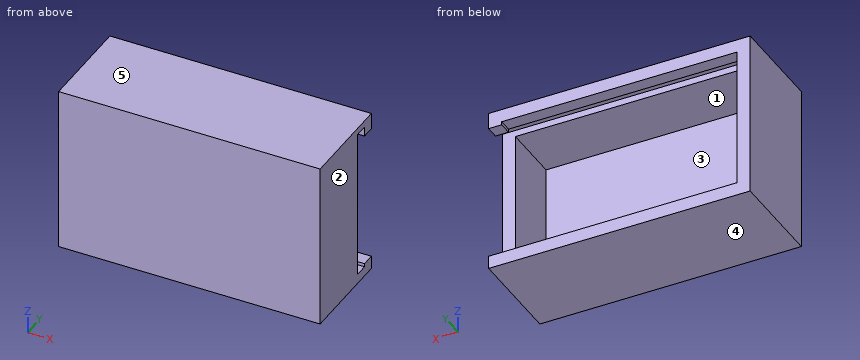
from build123d import *

# Parameters (mm, degrees)
SKETCH1_W           = 40
SKETCH1_H           = 25.5
BOSS_EXTRUDE1_DEPTH = 15
SHELL1_T            = -2
SKETCH2_W           = 21
SKETCH2_H           = 4
CUT_EXTRUDE1_DEPTH  = 2
SKETCH3_W           = 23.01
SKETCH3_H           = 2
CUT_EXTRUDE2_DEPTH  = 38


with BuildPart() as part:
    # Sketch1 → Boss-Extrude1 (new body)
    with BuildSketch(Plane(origin=(0, 0, 0), x_dir=(1, 0, 0), z_dir=(0, 1, 0))):
        Rectangle(SKETCH1_W, SKETCH1_H)
    extrude(amount=BOSS_EXTRUDE1_DEPTH)

    # Shell1
    shell1_openings = [part.faces().sort_by_distance(p)[0] for p in [
        (0, 15, 0),
    ]]
    offset(amount=SHELL1_T, openings=shell1_openings, kind=Kind.INTERSECTION)

    # Sketch2 → Cut-Extrude1 (cut)
    with BuildSketch(Plane(origin=(20, 0, 0), x_dir=(0, 0, -1), z_dir=(1, 0, 0))):
        with Locations((0.25, 13)):
            Rectangle(SKETCH2_W, SKETCH2_H)
    extrude(amount=-CUT_EXTRUDE1_DEPTH, mode=Mode.SUBTRACT)

    # Sketch3 → Cut-Extrude2 (cut)
    with BuildSketch(Plane(origin=(20, 0, 0), x_dir=(0, 0, -1), z_dir=(1, 0, 0))):
        with Locations((-0.245, 12)):
            Rectangle(SKETCH3_W, SKETCH3_H)
    extrude(amount=-CUT_EXTRUDE2_DEPTH, mode=Mode.SUBTRACT)


solid = part.part
Part model, mm, in its own coordinate system. Face numbers are marked on the shaded views. A direction names the side the tool comes from. Coordinates: 2 decimals unless noted, no trailing zeros. Loops run counter-clockwise (first coordinate to the right, second up) from the corner with the lowest first, then second, coordinate; pieces in that order, holes last. Notation, with made-up numbers: (-37.5, -14.75) -> (-18.5, -14.75) arc R20 cw to (-18.5, 5.25) -> close; hole circle Ø2 at (-28.75, 38). An arc over 180 degrees is marked (long way). Use a Markdown table: item, result. Add a question column.
Item 1: Band-saw the part on A-A on y = 6.25. Write the cut outline in (x, z), plus the area to 3 significant figures.
Item 2: Pull direction Z, two halves, no side cores. Call the marked faces 3, 4 and 5: +Z half, -Z half, draft (parallel to the pull), parting line (faces both ways), or undercut.
Item 3: Band-saw the part on C-C on x = -15. Write the cut outline in (y, z), plus the area to 4 significant figures.
Item 4: Which spindle directions (+Z, -Z, +X, -X, +Y, -Y) get a long thin tool onto all of the face, cutting with end or side? Do the marked faces 1 and 2. Say none if no direction does.
Item 5: Flat gauge pin, fed straight in: P1, Ø7, axis at x = -6, z = -3.5, coming from the +Y side. Where does the tip first touch, or does it go through?
Item 6: Probe probe 1 along Z at (x, y) = (3.5, 4); probe 2 along X at (y, z) = (3.75, 5); probe 3 along Y at (x, z) = (10.5, -9.75). List the from-to ranges inside material, lowest first.
Item 7: Band-saw the part on B-B on z = 2. Write the cut outline in (x, y), plus the area to 3 significant figures.
Geometry says:
| question | item | result |
|---|---|---|
| 1 | outline | (-20, -12.75) -> (20, -12.75) -> (20, 12.75) -> (-20, 12.75) -> close; hole (-18, -10.75) -> (18, -10.75) -> (18, 10.75) -> (-18, 10.75) -> close |
| 1 | area | 246 mm² |
| 2 | face 3 | undercut |
| 2 | face 4 | -Z half |
| 2 | face 5 | +Z half |
| 3 | outline | (0, -12.75) -> (15, -12.75) -> (15, -10.75) -> (13, -10.75) -> (13, -11.26) -> (11, -11.26) -> (11, -10.75) -> (2, -10.75) -> (2, 10.75) -> (11, 10.75) -> (11, 11.75) -> (13, 11.75) -> (13, 10.75) -> (15, 10.75) -> (15, 12.75) -> (0, 12.75) -> close |
| 3 | area | 100.0 mm² |
| 4 | face 1 | +Y |
| 4 | face 2 | +Z, -Z, +X, +Y, -Y |
| 5 | P1 | y = 2 |
| 6 | probe 1 | -12.75 to -10.75, 10.75 to 12.75 |
| 6 | probe 2 | -20 to -18, 18 to 20 |
| 6 | probe 3 | 0 to 2 |
| 7 | outline | (-20, 0) -> (20, 0) -> (20, 11) -> (18, 11) -> (18, 2) -> (-18, 2) -> (-18, 15) -> (-20, 15) -> close |
| 7 | area | 124 mm² |
